Verification items for this drawing (mm, ordinates from the low corner). Give positions to 0.01 mm unless a question says otherwise; leave off trailing zeros. Order: outer loops, then holes, each group sorted by start corner. A loop starts at its lowest first (then second) coordinate and runs counter-clockwise, first axis right, second up. Notation, with made-up numbers: (16, 42.25) -> (33, 42.25) arc R19 ccw to (33, 55.25) -> close; hole circle Ø3 at (-28, 35). An arc over 180 degrees is marked (long way). One line per question, with ' | ' between items.
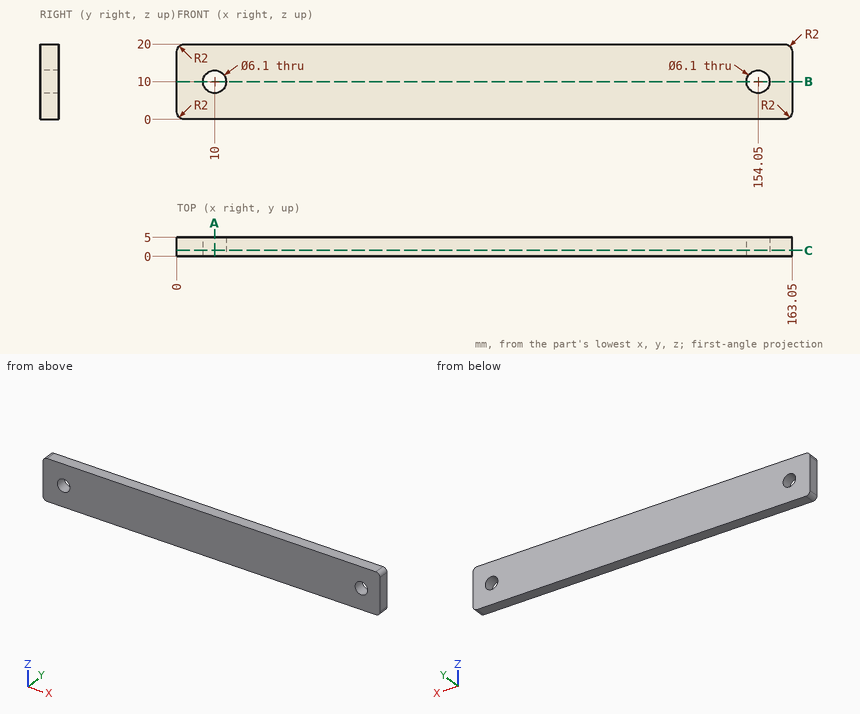
Q1. Section check C-C (y = 1.55). Enter the section's corners in (x, z), and give its area (3 significant figures).
Result sheet:
outline: (0, 2) arc R2 ccw to (2, 0) -> (161.05, 0) arc R2 ccw to (163.05, 2) -> (163.05, 18) arc R2 ccw to (161.05, 20) -> (2, 20) arc R2 ccw to (0, 18) -> close; hole circle Ø6.1 at (10, 10); hole circle Ø6.1 at (154.05, 10) | area: 3,200 mm2
Q2. Thickness scan on line 1 (Z direction, x = 154.05, y = 2.3); line 2 (X direction, y = 1, z = 11.5); line 3 (X direction, y = 0.75, z = 7.75). Record the ranges inside material, lowest first.
Result sheet:
line 1: z = 0 to 6.95, 13.05 to 20 | line 2: x = 0 to 7.34, 12.66 to 151.39, 156.71 to 163.05 | line 3: x = 0 to 7.94, 12.06 to 151.99, 156.11 to 163.05
Q3. Section check B-B (z = 10). Enter the section's corners in (x, y), and give its area (3 significant figures).
Result sheet:
outline: (0, 0) -> (6.95, 0) -> (6.95, 5) -> (0, 5) -> close; (13.05, 0) -> (151, 0) -> (151, 5) -> (13.05, 5) -> close; (157.1, 0) -> (163.05, 0) -> (163.05, 5) -> (157.1, 5) -> close | area: 754 mm2
Q4. Section check A-A (x = 10). Enter the section's corners in (y, z), and give its area (3 significant figures).
Result sheet:
outline: (0, 0) -> (5, 0) -> (5, 6.95) -> (0, 6.95) -> close; (0, 13.05) -> (5, 13.05) -> (5, 20) -> (0, 20) -> close | area: 69.5 mm2
